Geometry: final body of the model. Coordinates: model frame, mm. Face numbers are marked on the shaded views. A direction names the side the tool comes from. Round coordinates to 2 decimals unless told otherwise and drop trailing zeros. Loops run counter-clockwise (first coordinate to the right, second up) from the corner with the lowest first, then second, coordinate; pieces in that order, holes last. Notation, with made-up numbers: (14, -38.5) - (49, -38.5) arc R28 cw to (49, -2.5) - close; hole circle Ø7 at (16.25, 41.5). An arc over 180 degrees is marked (long way). Use CSV: the item, a comma, the result in double quotes.
from build123d import *

# Parameters (mm, degrees)
SKETCH2_R               = 2.75
SKETCH2_R_2             = 2
BOSS_EXTRUDE1_DEPTH     = 5
CUT_EXTRUDE1_START      = 1.5
SKETCH4_R               = 5.75
CUT_EXTRUDE1_DEPTH      = 4.5
CUT_EXTRUDE2_START      = -5
SKETCH5_R               = 5.5
CUT_EXTRUDE2_DEPTH      = 2.8
CUT_EXTRUDE2_DEPTH_BACK = 2.8
SKETCH6_R               = 2
BOSS_EXTRUDE2_DEPTH     = 10


with BuildPart() as part:
    # Sketch2 → Boss-Extrude1 (new body, symmetric)
    with BuildSketch(Plane(origin=(0, 0, 0), x_dir=(1, 0, 0), z_dir=(0, 1, 0))):
        with BuildLine():
            ThreePointArc((-11.219654399, -2.057358528), (-5.949237585, -8.991377869), (-1.50658351, -1.5))
            Line((-1.50658351, -1.5), (10, -1.5))
            Line((10, -1.5), (15, -5.195678453))
            Line((15, -5.195678453), (25, -1.5))
            Line((25, -1.5), (25, 3))
            Line((25, 3), (-21, 3))
            ThreePointArc((-21, 3), (-30, 0), (-21, -3))
            Line((-21, -3), (-20.25, -3))
            Line((-20.25, -3), (-11.219654399, -2.057358528))
        make_face()
        with Locations((-6.25, -3.75)):
            Circle(SKETCH2_R, mode=Mode.SUBTRACT)
        with Locations((-25, 0)):
            Circle(SKETCH2_R_2, mode=Mode.SUBTRACT)
    extrude(amount=BOSS_EXTRUDE1_DEPTH, both=True)

    # Sketch4 → Cut-Extrude1 (cut, through all)
    with BuildSketch(Plane(origin=(0, 0, 0), x_dir=(1, 0, 0), z_dir=(0, 1, 0)).offset(CUT_EXTRUDE1_START)):
        with Locations((-6.25, -3.75)):
            Circle(SKETCH4_R)
    cut_extrude1 = extrude(amount=CUT_EXTRUDE1_DEPTH, mode=Mode.SUBTRACT)

    # Sketch5 → Cut-Extrude2 (cut, two sides)
    with BuildSketch(Plane(origin=(0, 5, 0), x_dir=(1, 0, 0), z_dir=(0, 1, 0)).offset(CUT_EXTRUDE2_START)) as cut_extrude2_sk:
        with Locations((-25, 0)):
            Circle(SKETCH5_R)
    extrude(amount=CUT_EXTRUDE2_DEPTH, mode=Mode.SUBTRACT)
    extrude(cut_extrude2_sk.sketch, amount=-CUT_EXTRUDE2_DEPTH_BACK, mode=Mode.SUBTRACT)

    # Mirror1: Cut-Extrude1 across plane
    add(cut_extrude1.mirror(Plane.ZX), mode=Mode.SUBTRACT)

    # Sketch6 → Boss-Extrude2 (add)
    with BuildSketch(Plane(origin=(0, 5, 0), x_dir=(1, 0, 0), z_dir=(0, 1, 0))):
        with Locations((-25, 0)):
            Circle(SKETCH6_R)
    extrude(amount=-BOSS_EXTRUDE2_DEPTH)


solid = part.part
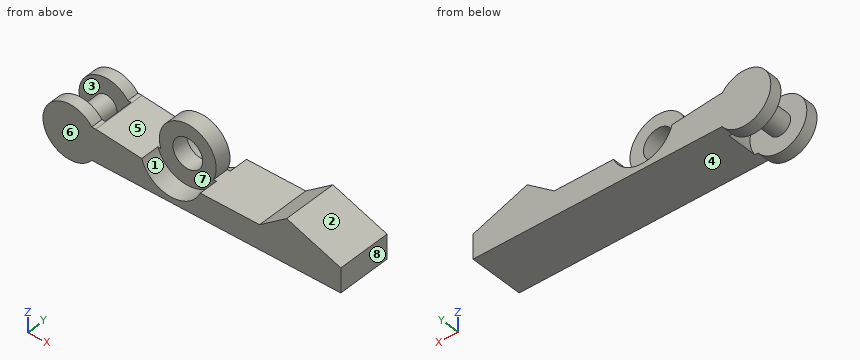
Item 1: Section A-A on y = -0.5. Return the cut outline in (x, z), plus the area to 3 significant figures.
Final values:
outline,"circle Ø4 at (-25, 0); (-20.39, -3) - (25, -3) - (25, 1.5) - (15, 5.2) - (10, 1.5) - (-1.51, 1.5) arc R5.25 ccw (long way) to (-11.22, 2.06) - (-20.25, 3) - (-20.39, 3) arc R5.5 cw to start; hole circle Ø5.5 at (-6.25, 3.75)"
area,"293 mm²"
Item 2: Section D-D on y = -3.75. Return the cut outline in (x, z).
Final values:
outline,"(-21, -3) - (25, -3) - (25, 1.5) - (15, 5.2) - (10, 1.5) - (-0.96, 1.5) arc R5.75 cw to (-11.76, 2.11) - (-20.25, 3) - (-21, 3) arc R5 ccw (long way) to start"
Item 3: Material intervals for line 1 (X direction, y = 2.5, z = -1.25); line 2 (Z direction, x = -6.25, y = 0.05); line 3 (Z direction, x = 7, y = 2.5), sorted ascending.
Final values:
line 1,"x = -26.56 to -23.44, -19.64 to -9.09, -3.41 to 25"
line 2,"z = -3 to 1, 6.5 to 9"
line 3,"z = -3 to 1.5"
Item 4: Section B-B on x = -6.25. Return the cut outline in (y, z).
Final values:
outline,"(-5, -3) - (5, -3) - (5, -2) - (1.5, -2) - (1.5, 1) - (-1.5, 1) - (-1.5, -2) - (-5, -2) - close; (-1.5, 6.5) - (1.5, 6.5) - (1.5, 9) - (-1.5, 9) - close"
Item 5: Reachability of the marked faces 1, 2, 3 and 4 from +Z, -Z, +X, -X, +Y, -Y: full face, straight path, thin tool, end or side. Return the list, or none.
Final values:
face 1,"+Z, -Y"
face 2,"+Z, +X, +Y, -Y"
face 3,"none"
face 4,"-Z, +X, +Y, -Y"
Item 6: Pin query (flat end, axial travel): P1, Ø5, axis at x = -8, y = -2.5, coming from the -Z side; P2, Ø3, axis at x = 6.5, y = 1, coming from the +Z side; P3, Ø7, axis at x = -6.25, z = 3.75, coming from the +Y side. Return the tip coordinate at first contact, or that it passes through.
Final values:
P1,"stops at z = -3"
P2,"stops at z = 1.5"
P3,"stops at y = 1.5"
Item 7: Section C-C on z = 0. Return the cut outline in (x, y), plus the area to 3 significant figures.
Final values:
outline,"(-30, -5) - (-10.61, -5) - (-10.61, -1.5) - (-1.89, -1.5) - (-1.89, -5) - (25, -5) - (25, 5) - (-1.89, 5) - (-1.89, 1.5) - (-10.61, 1.5) - (-10.61, 5) - (-30, 5) - (-30, 2.8) - (-27, 2.8) - (-27, -2.8) - (-30, -2.8) - close; hole (-23, -2.8) - (-19.5, -2.8) - (-19.5, 2.8) - (-23, 2.8) - close"
area,"453 mm²"
Item 8: Mould query, pull axis X, two halves, no side actions, for the marked faces 5, 6, 7 and 8. Classes: released by +X, released by -X, zero draft, split by the parting line, or undercut.
Final values:
face 5,"undercut"
face 6,"zero draft"
face 7,"undercut"
face 8,"released by +X"
